```python
from build123d import *

# Parameters (mm, degrees)
SKETCH_2_R               = 100
EXTRUDE_1_DEPTH          = 27
CUT_EXTRUDE_1_DEPTH      = 144.975692393
CUT_EXTRUDE_1_DEPTH_BACK = 10
SKETCH_2_8_R             = 41.5
CUT_EXTRUDE_4_DEPTH      = 140.593830451
CUT_EXTRUDE_7_DEPTH      = 140.593830451
CUT_EXTRUDE_7_DEPTH_BACK = 10
SKETCH_2_11_R            = 2.1
CUT_EXTRUDE_8_DEPTH      = 140.593830451
CUT_EXTRUDE_8_DEPTH_BACK = 140.593830451
SKETCH_6_R               = 1.6
SKETCH_6_R_2             = 1.5
CUT_EXTRUDE_9_DEPTH      = 140.593830451
CUT_EXTRUDE_9_DEPTH_BACK = 140.593830451
SKETCH_7_R               = 2.5


with BuildPart() as part:
    # Sketch 2 → Extrude 1 (new body)
    with BuildSketch(Plane(origin=(0, 0, 0), x_dir=(1, 0, 0), z_dir=(0, 1, 0))):
        with Locations(Location((0, 0, 0), (0, 0, 270))):
            Circle(SKETCH_2_R)
    extrude(amount=EXTRUDE_1_DEPTH)

    # Sketch 2_5 → Cut-Extrude 1 (cut, two sides: drawn at the far end of the back side and taken through both)
    with BuildSketch(Plane(origin=(0, 0, 0), x_dir=(1, 0, 0), z_dir=(0, 1, 0)).offset(-CUT_EXTRUDE_1_DEPTH_BACK)):
        with BuildLine():
            Line((-74.428393142, 35.25), (-93.581181335, 35.25))
            ThreePointArc((-93.581181335, 35.25), (-99.86554004, -5.184005444), (-89.428393142, -44.75))
            Line((-89.428393142, -44.75), (-74.428393142, -44.75))
            Line((-74.428393142, -44.75), (-74.428393142, -20.75))
            Line((-74.428393142, -20.75), (-74.428393142, 35.25))
        make_face()
        with BuildLine():
            Line((93.581181335, 35.25), (74.428393142, 35.25))
            Line((74.428393142, 35.25), (74.428393142, -20.75))
            Line((74.428393142, -20.75), (74.428393142, -44.75))
            Line((74.428393142, -44.75), (89.428393142, -44.75))
            ThreePointArc((89.428393142, -44.75), (97.321218946, -22.990875209), (100, 0))
            ThreePointArc((100, 0), (98.382209097, 17.914824399), (93.581181335, 35.25))
        make_face()
    extrude(amount=CUT_EXTRUDE_1_DEPTH + CUT_EXTRUDE_1_DEPTH_BACK, mode=Mode.SUBTRACT)

    # Sketch 2_8 → Cut-Extrude 4 (cut, through all)
    with BuildSketch(Plane(origin=(0, 0, 0), x_dir=(1, 0, 0), z_dir=(0, 1, 0))):
        with Locations(Location((0, 12.743545883, 0), (0, 0, 270))):
            Circle(SKETCH_2_8_R)
    extrude(amount=CUT_EXTRUDE_4_DEPTH, mode=Mode.SUBTRACT)

    # Sketch 2_11 → Cut-Extrude 7 (cut, two sides: drawn at the far end of the back side and taken through both)
    with BuildSketch(Plane(origin=(0, 0, 0), x_dir=(1, 0, 0), z_dir=(0, 1, 0)).offset(-CUT_EXTRUDE_7_DEPTH_BACK)):
        with Locations(Location((0, -45, 0), (0, 0, 270))):
            Circle(SKETCH_2_11_R)
        with Locations(Location((0, -88.65, 0), (0, 0, 270))):
            Circle(SKETCH_2_11_R)
    extrude(amount=CUT_EXTRUDE_7_DEPTH + CUT_EXTRUDE_7_DEPTH_BACK, mode=Mode.SUBTRACT)

    # Sketch 6 → Cut-Extrude 8 (cut, two sides: drawn at the far end of the back side and taken through both)
    with BuildSketch(Plane(origin=(0, 27, 0), x_dir=(1, 0, 0), z_dir=(0, 1, 0)).offset(-CUT_EXTRUDE_8_DEPTH_BACK)):
        with BuildLine():
            Line((-58.41813564, -34.974946877), (-58.41813564, -33.374946877))
            Line((-58.41813564, -33.374946877), (-56.81813564, -33.374946877))
            ThreePointArc((-56.81813564, -33.374946877), (-59.54950649, -32.243576027), (-58.41813564, -34.974946877))
        make_face()
        with BuildLine():
            Line((-56.81813564, -33.374946877), (-58.41813564, -33.374946877))
            Line((-58.41813564, -33.374946877), (-58.41813564, -34.974946877))
            ThreePointArc((-58.41813564, -34.974946877), (-57.28676479, -34.506317727), (-56.81813564, -33.374946877))
        make_face()
        with BuildLine():
            ThreePointArc((-19.81813564, -33.374946877), (-21.41813564, -31.774946877), (-23.01813564, -33.374946877))
            Line((-23.01813564, -33.374946877), (-21.41813564, -33.374946877))
            Line((-21.41813564, -33.374946877), (-21.41813564, -34.974946877))
            ThreePointArc((-21.41813564, -34.974946877), (-20.28676479, -34.506317727), (-19.81813564, -33.374946877))
        make_face()
        with BuildLine():
            Line((-21.41813564, -33.374946877), (-23.01813564, -33.374946877))
            ThreePointArc((-23.01813564, -33.374946877), (-22.54950649, -34.506317727), (-21.41813564, -34.974946877))
            Line((-21.41813564, -34.974946877), (-21.41813564, -33.374946877))
        make_face()
        with BuildLine():
            ThreePointArc((-56.81813564, -70.374946877), (-57.28676479, -69.243576027), (-58.41813564, -68.774946877))
            Line((-58.41813564, -68.774946877), (-58.41813564, -70.374946877))
            Line((-58.41813564, -70.374946877), (-56.81813564, -70.374946877))
        make_face()
        with BuildLine():
            Line((-58.41813564, -70.374946877), (-58.41813564, -68.774946877))
            ThreePointArc((-58.41813564, -68.774946877), (-59.54950649, -71.506317727), (-56.81813564, -70.374946877))
            Line((-56.81813564, -70.374946877), (-58.41813564, -70.374946877))
        make_face()
        with Locations(Location((-21.41813564, -70.374946877, 0), (0, 0, 270))):
            Circle(SKETCH_6_R)
        with Locations(Location((-70, -55, 0), (0, 0, 270))):
            Circle(SKETCH_6_R_2)
        with Locations(Location((-70, 55, 0), (0, 0, 270))):
            Circle(SKETCH_6_R_2)
        with Locations(Location((70, 55, 0), (0, 0, 270))):
            Circle(SKETCH_6_R_2)
        with Locations(Location((70, -55, 0), (0, 0, 270))):
            Circle(SKETCH_6_R_2)
    extrude(amount=CUT_EXTRUDE_8_DEPTH + CUT_EXTRUDE_8_DEPTH_BACK, mode=Mode.SUBTRACT)

    # Sketch 7 → Cut-Extrude 9 (cut, two sides: drawn at the far end of the back side and taken through both)
    with BuildSketch(Plane(origin=(0, 27, 0), x_dir=(1, 0, 0), z_dir=(0, 1, 0)).offset(-CUT_EXTRUDE_9_DEPTH_BACK)):
        with Locations(Location((-26.5, 72.61491789, 0), (0, 0, 270))):
            Circle(SKETCH_7_R)
        with Locations(Location((26.5, 72.61491789, 0), (0, 0, 270))):
            Circle(SKETCH_7_R)
    extrude(amount=CUT_EXTRUDE_9_DEPTH + CUT_EXTRUDE_9_DEPTH_BACK, mode=Mode.SUBTRACT)


solid = part.part
```
Geometry: final body of the model. Coordinates: model frame, mm. A direction names the side the tool comes from. Round coordinates to 2 decimals unless told otherwise and drop trailing zeros. Order: outer loops, then holes, each group sorted by start corner. A loop starts at its lowest first (then second) coordinate and runs counter-clockwise, first axis right, second up. Notation, with made-up numbers: M 49.5,37.5 L 74.5,37.5 A16 cw 74.5,51.5 Z; hole C -6.75,68.5 d4. An arc over 180 degrees is marked long. One line per item, written item: value.
(1) Cut plane B-B (x = 32.5). Return the cut outline in (y, z).
Result sheet:
outline: M 0,-94.57 L 27,-94.57 L 27,-38.55 L 0,-38.55 Z; M 0,13.06 L 27,13.06 L 27,94.57 L 0,94.57 Z
(2) Pull-direction query (X, two-part tool) for faces 4 (the cylindrical face through (-0.8, 13.31, 46.94)), 5 (the cylindrical face through (1.695, 13.311, -99.986)), 6 (the flat face through (84, 13, -35.25)); classes: pulls with the +X half, pulls with the -X half, needs draft (parallel to the pull), parting line crosses it, or undercut.
Result sheet:
face 4: undercut
face 5: parting line crosses it
face 6: needs draft
(3) Pin query (flat end, axial travel): P1, Ø3, axis at x = 18.5, y = 3.5, coming from the -Z side; P2, Ø9.5, axis at x = -81.5, y = 7.5, coming from the +Z side; P3, Ø13.5, axis at y = 17.5, z = 16.5, coming from the -X side; P4, Ø5, axis at x = 70, z = -55, coming from the -Y side. Return the tip coordinate at first contact, or that it passes through.
Result sheet:
P1: z = -98.54
P2: z = 64.1
P3: x = -74.43
P4: y = 0
(4) Line query: probe 1 along X at (y, z) = (10.25, -55); probe 2 along Z at (x, y) = (-57, 17.75); probe 3 along X at (y, z) = (6, 7.5). Output: solid intervals per line, ascending. Write a range as [from, to].
Result sheet:
probe 1: [-83.52, -71.5], [-68.5, 68.5], [71.5, 83.52]
probe 2: [-82.16, 32.63], [34.12, 69.63], [71.12, 82.16]
probe 3: [-74.43, -36.23], [36.23, 74.43]
(5) Cut plane A-A (y = 8.25). Give the number of separate pieces and of enclosed holes in the cut face, and give its area (3 significant figures).
Result sheet:
separate pieces: 1
enclosed holes: 13
area: 22,200 mm2
(6) Cut plane C-C (x = -26.5). Return the cut outline in (y, z).
Result sheet:
outline: M 0,-96.42 L 27,-96.42 L 27,-75.11 L 0,-75.11 Z; M 0,-70.11 L 27,-70.11 L 27,-44.68 L 0,-44.68 Z; M 0,19.19 L 27,19.19 L 27,96.42 L 0,96.42 Z
(7) Cut plane D-D (x = 13.5). Return the cut outline in (y, z), and give its area (3 significant figures).
Result sheet:
outline: M 0,-99.08 L 27,-99.08 L 27,-51.99 L 0,-51.99 Z; M 0,26.5 L 27,26.5 L 27,99.08 L 0,99.08 Z
area: 3,230 mm2
(8) Reachability of faces 1 (the cylindrical face through (27.25, 13.31, -70.23)), 2 (the flat face through (-84, 13, -35.25)), 3 (the flat face through (74.428, 13, 4)) from +Z, -Z, +X, -X, +Y, -Y: full face, straight path, thin tool, end or side. Return the list, or none.
Result sheet:
face 1: +Y, -Y
face 2: -X, +Y, -Y
face 3: +X, +Y, -Y
